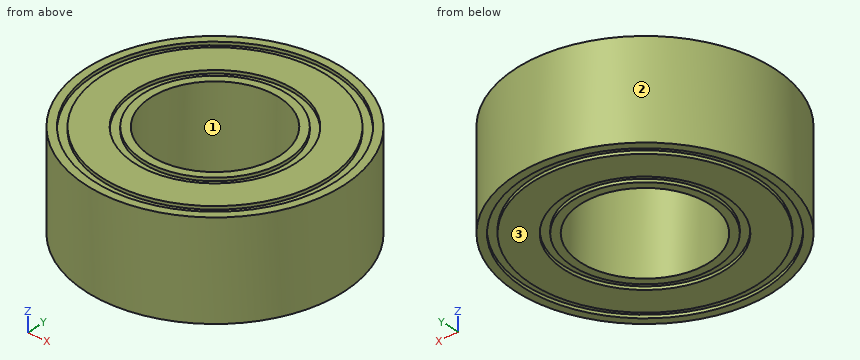
from build123d import *

# Parameters (mm, degrees)
SKETCH_1_R          = 4
SKETCH_1_R_2        = 2
EXTRUDE_1_DEPTH     = 3
SKETCH_2_R          = 3.75
SKETCH_2_R_2        = 3.5
SKETCH_2_R_3        = 2.5
SKETCH_2_R_4        = 2.25
CUT_EXTRUDE_1_DEPTH = 0.1
CUT_EXTRUDE_START   = -0.1
SKETCH_3_R          = 3.75
SKETCH_3_R_2        = 3.5
SKETCH_3_R_3        = 2.5
SKETCH_3_R_4        = 2.25
CUT_EXTRUDE_2_DEPTH = 0.1


with BuildPart() as part:
    # 草图1 → 凸台-拉伸1 (new body)
    with BuildSketch(Plane.XY):
        Circle(SKETCH_1_R)
        Circle(SKETCH_1_R_2, mode=Mode.SUBTRACT)
    extrude(amount=EXTRUDE_1_DEPTH)

    # 草图2 → 切除-拉伸1 (cut)
    # profile 1 of 2: a face of its own
    with BuildSketch(Plane.XY.offset(3)):
        Circle(SKETCH_2_R)
        Circle(SKETCH_2_R_2, mode=Mode.SUBTRACT)
    # profile 2 of 2: a face of its own
    with BuildSketch(Plane.XY.offset(3)):
        Circle(SKETCH_2_R_3)
        Circle(SKETCH_2_R_4, mode=Mode.SUBTRACT)
    extrude(amount=-CUT_EXTRUDE_1_DEPTH, mode=Mode.SUBTRACT)

    # 草图3 → 切除-拉伸2 (cut)
    # profile 1 of 2: a face of its own
    with BuildSketch(Plane(origin=(0, 0, 0), x_dir=(-1, 0, 0), z_dir=(0, 0, -1)).offset(CUT_EXTRUDE_START)):
        with Locations(Location((0, 0, 0), (0, 0, 180))):
            Circle(SKETCH_3_R)
        with Locations(Location((0, 0, 0), (0, 0, 180))):
            Circle(SKETCH_3_R_2, mode=Mode.SUBTRACT)
    # profile 2 of 2: a face of its own
    with BuildSketch(Plane(origin=(0, 0, 0), x_dir=(-1, 0, 0), z_dir=(0, 0, -1)).offset(CUT_EXTRUDE_START)):
        with Locations(Location((0, 0, 0), (0, 0, 180))):
            Circle(SKETCH_3_R_3)
        with Locations(Location((0, 0, 0), (0, 0, 180))):
            Circle(SKETCH_3_R_4, mode=Mode.SUBTRACT)
    extrude(amount=CUT_EXTRUDE_2_DEPTH, mode=Mode.SUBTRACT)


solid = part.part
The listing builds one solid part. Answer for the finished solid, in the listing's coordinates (mm). Face numbers are marked on the shaded views. Coordinates: 2 decimals unless noted, no trailing zeros. Write each loop counter-clockwise with the first axis right and the second up, starting at its lowest first coordinate (ties: lowest second). Pieces come first, ordered by that corner, then holes. Notation, with made-up numbers: M 33.25,-18 L 64.25,-18 A27 cw 64.25,5 Z; hole C -6.5,84.25 d2. An arc over 180 degrees is marked long. Put each result on its own line as item: value. Start each with the question number.
1. A cutting plane is placed at C-C on x = -3. Write down the section's boundary in (y, z).
2. Flat-ended cylindrical pins translate along their axes: P1, Ø1, axis at x = 1, z = 1, coming from the +Y side; P2, Ø1.5, axis at y = 3, z = 2.5, coming from the +X side; P3, Ø1.5, axis at x = -0.5, y = -1, coming from the +Z side. Find the tip coordinate at first contact, or state that the pin passes through.
3. A cutting plane is placed at B-B on y = -2.75. Write down the section's boundary in (x, z).
4. For a pull along X with two mould halves and no side action, classify the marked faces 1, 2 and 3 as pulls with the +X half, pulls with the -X half, needs draft (parallel to the pull), parting line crosses it, or undercut.
5. Consider line 1 (Y direction, x = 0, z = 0.05); line 2 (Y direction, x = 0, z = 1.2); line 3 (Z direction, x = 2.5, y = -2.75). Determine where each line is inside the solid, lowest interval first. Write a range as from..to.
6. A cutting plane is placed at A-A on z = 0.4. Write down the section's boundary in (x, y).
Resolved:
1. outline: M -2.65,0 L -2.25,0 L -2.25,0.1 L -1.8,0.1 L -1.8,0 L 1.8,0 L 1.8,0.1 L 2.25,0.1 L 2.25,0 L 2.65,0 L 2.65,3 L 2.25,3 L 2.25,2.9 L 1.8,2.9 L 1.8,3 L -1.8,3 L -1.8,2.9 L -2.25,2.9 L -2.25,3 L -2.65,3 Z
2. P1: stops at y = 3.97
2. P2: stops at x = 3.31
2. P3: passes through
3. outline: M -2.9,0 L -2.55,0 L -2.55,0.1 L -2.17,0.1 L -2.17,0 L 2.17,0 L 2.17,0.1 L 2.55,0.1 L 2.55,0 L 2.9,0 L 2.9,3 L 2.55,3 L 2.55,2.9 L 2.17,2.9 L 2.17,3 L -2.17,3 L -2.17,2.9 L -2.55,2.9 L -2.55,3 L -2.9,3 Z
4. face 1: undercut
4. face 2: parting line crosses it
4. face 3: needs draft
5. line 1: y = -4..-3.75, -3.5..-2.5, -2.25..-2, 2..2.25, 2.5..3.5, 3.75..4
5. line 2: y = -4..-2, 2..4
5. line 3: z = 0.1..2.9
6. outline: C 0,0 d8; hole C 0,0 d4
